The model under review builds one solid part; all positions refer to its coordinate system, in mm. A direction names the side the tool comes from. Coordinates: 2 decimals unless noted, no trailing zeros. Loops run counter-clockwise (first coordinate to the right, second up) from the corner with the lowest first, then second, coordinate; pieces in that order, holes last. Notation, with made-up numbers: (51, -34) - (67, -34) arc R21 cw to (67, -7) - close; hole circle Ø10 at (74, 60.5). An arc over 180 degrees is marked (long way). Use a Markdown table: item, result. Add a question column.
1) The part is to be moulded in two halves that separate along Z. For faces 1 (the cylindrical face through (17.084, 9.014, 3.794)), 2 (the flat face through (0, 0, 0)), 3 (the cylindrical face through (3.47, 3.55, 6.08)), say which applies: pulls with the +Z half, pulls with the -Z half, needs draft (parallel to the pull), parting line crosses it, or undercut.
2) Add section A-A, the plane y = 3. Give the boundary of the cut face in (x, z), and give its area (3 significant figures).
3) Add section C-C, the plane z = 0. Give the boundary of the cut face in (x, y), and give its area (3 significant figures).
4) For faces 4 (the flat face through (5, 8, 17)), 5 (the cylindrical face through (5.2, 3.55, -2.99)), 6 (the cylindrical face through (5.584, 8.521, 7.266)), list the 3-axis set-ups (+Z, -Z, +X, -X, +Y, -Y) from which the entire face can be reached by the end or side of a thin tool; tool diameter is ignored.
5) Clearance check with flat-ended pins moving along their axes: pin 1 (4 mm diameter, centred on x = 7.07, z = 7.07, fed in from -Y); pin 2 (6 mm diameter, centred on y = 9, z = 5.5, fed in from -X); pin 3 (1 mm diameter, centred on y = 4.5, z = 1.5, fed in from +X). State where each tip first meets the part, or that it passes through.
6) To check wall thickness, follow L1, parallel to X at y = 4, z = 5; L2, parallel to Z at x = 3, y = 2.25; L3, parallel to X at y = 8.5, z = -8. State the ranges of each line that lie inside material, in increasing order. Write a range as [from, to].
7) Add section D-D, the plane x = -12. Give the boundary of the cut face in (y, z), and give its area (3 significant figures).
8) Add section B-B, the plane x = 0. Give the boundary of the cut face in (y, z).
```python
from build123d import *

# Parameters (mm, degrees)
SKETCH3_R          = 1.5
CUT_EXTRUDE1_DEPTH = 37.742346142
CIRPATTERN1_COUNT  = 4
CUT_EXTRUDE2_START = -7
CUT_EXTRUDE2_DEPTH = 7
CIRPATTERN2_COUNT  = 6


with BuildPart() as part:
    # Sketch2 → Revolve1 (revolve)
    with BuildSketch(Plane.XY, mode=Mode.PRIVATE) as revolve1_sk:
        Polygon((0, 0), (7, 0), (7, 7), (24, 7), (24, 0), (25, 0), (25, 8), (17.5, 8), (17.5, 10), (0, 10), align=None)
    revolve(revolve1_sk.sketch.rotate(Axis((0, 0, 0), (0, 1, 0)), 90), axis=Axis((0, 0, 0), (0, 1, 0)))

    # Sketch3 → Cut-Extrude1 (cut, through all)
    with BuildSketch(Plane(origin=(0, 10, 0), x_dir=(1, 0, 0), z_dir=(0, 1, 0))):
        with Locations(Location((-7.071067812, 7.071067812, 0), (0, 0, 270))):
            Circle(SKETCH3_R)
    cut_extrude1 = extrude(amount=-CUT_EXTRUDE1_DEPTH, mode=Mode.SUBTRACT)

    # CirPattern1: Cut-Extrude1 ×4 about axis
    cirpattern1_axis = Axis((0, 0, 0), (0, 1, 0))
    for i in range(1, CIRPATTERN1_COUNT):
        add(cut_extrude1.rotate(cirpattern1_axis, i * 360 / CIRPATTERN1_COUNT), mode=Mode.SUBTRACT)

    # Sketch4 → Cut-Extrude2 (cut)
    with BuildSketch(Plane.XZ.offset(CUT_EXTRUDE2_START)):
        with BuildLine():
            Line((-1.215537244, 6.893654271), (-1.041889066, 5.908846518))
            ThreePointArc((-1.041889066, 5.908846518), (0, 6), (1.041889066, 5.908846518))
            Line((1.041889066, 5.908846518), (1.215537244, 6.893654271))
            ThreePointArc((1.215537244, 6.893654271), (0, 7), (-1.215537244, 6.893654271))
        make_face()
    cut_extrude2 = extrude(amount=CUT_EXTRUDE2_DEPTH, mode=Mode.SUBTRACT)

    # CirPattern2: Cut-Extrude2 ×6 about axis
    cirpattern2_axis = Axis((0, 0, 0), (0, 1, 0))
    for i in range(1, CIRPATTERN2_COUNT):
        add(cut_extrude2.rotate(cirpattern2_axis, i * 360 / CIRPATTERN2_COUNT), mode=Mode.SUBTRACT)


solid = part.part
```
From the geometry:
| question | item | result |
|---|---|---|
| 1 | face 1 | parting line crosses it |
| 1 | face 2 | needs draft |
| 1 | face 3 | undercut |
| 2 | outline | circle Ø50 at (0, 0); (-6.58, -2.39) - (-5.64, -2.05) arc R6 ccw to (-4.6, -3.86) - (-5.36, -4.5) arc R7 ccw to (-1.22, -6.89) - (-1.04, -5.91) arc R6 ccw to (1.04, -5.91) - (1.22, -6.89) arc R7 ccw to (5.36, -4.5) - (4.6, -3.86) arc R6 ccw to (5.64, -2.05) - (6.58, -2.39) arc R7 ccw to (6.58, 2.39) - (5.64, 2.05) arc R6 ccw to (4.6, 3.86) - (5.36, 4.5) arc R7 ccw to (1.22, 6.89) - (1.04, 5.91) arc R6 ccw to (-1.04, 5.91) - (-1.22, 6.89) arc R7 ccw to (-5.36, 4.5) - (-4.6, 3.86) arc R6 ccw to (-5.64, 2.05) - (-6.58, 2.39) arc R7 ccw to start; hole circle Ø48 at (0, 0) |
| 2 | area | 294 mm^2 |
| 3 | outline | (-25, 0) - (-24, 0) - (-24, 7) - (-7, 7) - (-7, 0) - (7, 0) - (7, 7) - (24, 7) - (24, 0) - (25, 0) - (25, 8) - (17.5, 8) - (17.5, 10) - (-17.5, 10) - (-17.5, 8) - (-25, 8) - close |
| 3 | area | 232 mm^2 |
| 4 | face 4 | +Y |
| 4 | face 5 | -Y |
| 4 | face 6 | +Y, -Y |
| 5 | pin 1 | stops at y = 7 |
| 5 | pin 2 | stops at x = -24.86 |
| 5 | pin 3 | stops at x = 24.98 |
| 6 | L1 | x = [-24.49, -23.47], [-4.9, 4.9], [23.47, 24.49] |
| 6 | L2 | z = [-24.82, -23.81], [-6.32, 6.32], [23.81, 24.82] |
| 6 | L3 | x = [-15.56, -8.25], [-5.89, 5.89], [8.25, 15.56] |
| 7 | outline | (0, -21.93) - (8, -21.93) - (8, -12.74) - (10, -12.74) - (10, 12.74) - (8, 12.74) - (8, 21.93) - (0, 21.93) - (0, 20.78) - (7, 20.78) - (7, -20.78) - (0, -20.78) - close |
| 7 | area | 111 mm^2 |
| 8 | outline | (0, -25) - (8, -25) - (8, -17.5) - (10, -17.5) - (10, 17.5) - (8, 17.5) - (8, 25) - (0, 25) - (0, 24) - (7, 24) - (7, 6) - (0, 6) - (0, -6) - (7, -6) - (7, -24) - (0, -24) - close |
